Here's how the part is built. I have some questions about the finished solid (model axes, mm). A direction names the side the tool comes from. Coordinates: 2 decimals unless noted, no trailing zeros. Loops run counter-clockwise (first coordinate to the right, second up) from the corner with the lowest first, then second, coordinate; pieces in that order, holes last. Notation, with made-up numbers: (34.5, 3.25) -> (69.5, 3.25) arc R5 ccw to (69.5, 8.25) -> close; hole circle Ø3 at (49, 86.5). An arc over 180 degrees is marked (long way). Answer as a JSON object with one key per item and string values. Group by question number.
Q1. On a 3-axis mill with a long thin cutter (end or side, diameter ignored), from which of +Z, -Z, +X, -X, +Y, -Y can I reach the whole of each face in a straight line? I mean faces 1 (the flat face through (0, 17, 2.5)), 2 (the cylindrical face through (0.867, 7.902, 3.905)), 3 (the flat face through (0, 0, 0)). Say none if no direction works.
Q2. I want a section at B-B on y = 7.75. Write out the boundary of the cut face in (x, z), then the cut area to 3 significant figures.
Q3. I'm going to push flat-ended pins straight in: pin 1 (3 mm diameter, centred on x = 0.5, y = 17.5, fed in from -Z); pin 2 (4 mm diameter, centred on x = -1.5, y = 4, fed in from -Z); pin 3 (4 mm diameter, centred on x = 1, y = 3, fed in from +Z). Where does each tip first touch, or does it pass through?
Q4. I want a section at A-A on x = 0. Write out the boundary of the cut face in (y, z).
Q5. Thinking about a two-plate mould opening in Z: for faces 4 (the conical face through (-1.03, 18.31, -4.63)), 5 (the flat face through (3, 15, 3)), 6 (the flat face through (-2.155, 16.935, 1.267)), which applies, released by +Z, released by -Z, zero draft, split by the parting line, or undercut?
Q6. I need wall thicknesses on line 1 (Z direction, x = 2.5, y = 14.75); line 2 (X direction, y = 7, z = -1); line 3 (Z direction, x = -0.25, y = 7.25). Which ranges of each line are inside material? Lowest first, please.
Autodesk Inventor part; units mm, degrees
ref_plane "Work Plane1" through (0, 19.4, 0) normal (0, 1, 0) x (1, 0, 0)
ref_plane "YZ Plane" through (0, 0, 0) normal (1, 0, 0) x (0, 1, 0)
ref_plane "XZ Plane" through (0, 0, 0) normal (0, 1, 0) x (-1, 0, 0)
sketch "Sketch1" plane through (0, 0, 0) normal (0, 1, 0) x (-1, 0, 0)
  circle A0 centre (0, 0) radius 4
  dimension "d0" = 8
extrude "Extrusion1" add sketch "Sketch1" along normal blind 15
chamfer "Chamfer1" distance 1 angle 45 1 edges at (4, 0, 0)
ref_plane "Work Plane1" through (0, 19.4, 0) normal (0, 1, 0) x (1, 0, 0)
thread "Thread1"
sketch "Sketch5" plane through (0, 15, 0) normal (0, 1, 0) x (1, 0, 0)
  circle A0 centre (0, 0) radius 7
  dimension "d17" = 14
sketch "Sketch6" plane through (0, 19.4, 0) normal (0, 1, 0) x (1, 0, 0)
  circle A0 centre (0, 0) radius 4
  dimension "d18" = 8
loft "Loft2" add profiles "Sketch5", "Sketch6"
fillet "Fillet1" radius 2 1 edges at (-4, 19.4, 0)
sketch "Sketch7" plane through (0, 19.4, 0) normal (0, 1, 0) x (1, 0, 0)
  line L0 (2.8868, 0) -> (1.4434, -2.5)
  line L1 (1.4434, -2.5) -> (-1.4434, -2.5)
  line L2 (-1.4434, -2.5) -> (-2.8868, 0)
  line L3 (-2.8868, 0) -> (-1.4434, 2.5)
  line L4 (-1.4434, 2.5) -> (1.4434, 2.5)
  line L5 (1.4434, 2.5) -> (2.8868, 0)
  point P0 (0, 0)
  point P1 (0, 0)
  dimension "d24" = 5
extrude "Extrusion3" cut sketch "Sketch7" against normal blind 5
properties part number "M8x15"
Result set:
{
 "1": {"face 1": "+Y", "face 2": "-Y", "face 3": "+Z, -Z, +X, -X, -Y"},
 "2": {"outline": "circle Ø8 at (0, 0)", "area": "50.3 mm²"},
 "3": {"pin 1": "stops at z = -6.3", "pin 2": "stops at z = -4", "pin 3": "stops at z = 4"},
 "4": {"outline": "(0, -3) -> (1, -4) -> (15, -4) -> (15, -7) -> (18.53, -4.6) arc R2 ccw to (19.4, -2.94) -> (19.4, -2.5) -> (14.4, -2.5) -> (14.4, 2.5) -> (19.4, 2.5) -> (19.4, 2.94) arc R2 ccw to (18.53, 4.6) -> (15, 7) -> (15, 4) -> (1, 4) -> (0, 3) -> close"},
 "5": {"face 4": "split by the parting line", "face 5": "zero draft", "face 6": "undercut"},
 "6": {"line 1": "z = -3.12 to -0.67, 0.67 to 3.12", "line 2": "x = -3.87 to 3.87", "line 3": "z = -3.99 to 3.99"}
}
